Design review of the part built by this model. Coordinates are the model's own, in mm. Coordinates: 2 decimals unless noted, no trailing zeros. Write each loop counter-clockwise with the first axis right and the second up, starting at its lowest first coordinate (ties: lowest second). Pieces come first, ordered by that corner, then holes. Notation, with made-up numbers: (46, 1.5) -> (61, 1.5) arc R31 ccw to (61, 28.5) -> close; hole circle Ø4 at (39.25, -26). An arc over 180 degrees is marked (long way). One line per question, with ' | ' between items. Start each with the question number.
Q1. Wall thickness on probe 1 along X at (y, z) = (87, 77.5); probe 2 along Y at (x, z) = (230, 255): over which ranges is each line inside the solid? List them lowest first.
Q2. Add section C-C on z = 242. State the section outline as (x, y) points.
Q3. For P1, Ø8, axis at y = 140.5, z = -215, coming from the +X side, flat-tipped, find the tip position at first contact; note if it passes through.
Q4. Add section A-A on x = 311.5. State the section outline as (y, z) points.
Q5. Add section D-D on y = 129. State the section outline as (x, z) points, and give its area (3 significant figures).
Q6. Add section B-B on z = 115. State the section outline as (x, y) points, and give its area (3 significant figures).
from build123d import *

# Parameters (mm, degrees)
SKETCH1_W           = 1416.83235241
SKETCH1_H           = 579.478309122
SKETCH1_W_2         = 1270
SKETCH1_H_2         = 434.999892
BOSS_EXTRUDE1_DEPTH = 2.54
SKETCH2_W           = 73.416176205
SKETCH2_H           = 579.478309122
BOSS_EXTRUDE2_DEPTH = 327.9394
SKETCH3_W           = 76.2
SKETCH3_H           = 25.4
BOSS_EXTRUDE3_DEPTH = 299.9994
SKETCH4_W           = 73.416176205
SKETCH4_H           = 579.478309122
BOSS_EXTRUDE4_DEPTH = 149.999954
SKETCH5_W           = 76.2
SKETCH5_H           = 25.4
BOSS_EXTRUDE5_DEPTH = 299.72


with BuildPart() as part:
    # Sketch1 → Boss-Extrude1 (new body)
    with BuildSketch(Plane(origin=(0, 0, 0), x_dir=(1, 0, 0), z_dir=(0, 1, 0))):
        Rectangle(SKETCH1_W, SKETCH1_H)
        Rectangle(SKETCH1_W_2, SKETCH1_H_2, mode=Mode.SUBTRACT)
    extrude(amount=BOSS_EXTRUDE1_DEPTH)

    # Sketch2 → Boss-Extrude2 (add)
    with BuildSketch(Plane.XZ):
        with Locations((-671.708088103, 0)):
            Rectangle(SKETCH2_W, SKETCH2_H)
    extrude(amount=-BOSS_EXTRUDE2_DEPTH)

    # Sketch3 → Boss-Extrude3 (add)
    with BuildSketch(Plane(origin=(-635, 0, 0), x_dir=(0, 0, -1), z_dir=(1, 0, 0))):
        with Locations((-251.639154561, 315.2394)):
            Rectangle(SKETCH3_W, SKETCH3_H)
        with Locations((251.639154561, 315.2394)):
            Rectangle(SKETCH3_W, SKETCH3_H)
    extrude(amount=BOSS_EXTRUDE3_DEPTH)

    # Sketch4 → Boss-Extrude4 (add)
    with BuildSketch(Plane(origin=(0, 327.9394, 0), x_dir=(1, 0, 0), z_dir=(0, 1, 0))):
        with Locations((-671.708088103, 0)):
            Rectangle(SKETCH4_W, SKETCH4_H)
    extrude(amount=BOSS_EXTRUDE4_DEPTH)

    # Sketch5 → Boss-Extrude5 (add)
    with BuildSketch(Plane(origin=(-635, 0, 0), x_dir=(0, 0, -1), z_dir=(1, 0, 0))):
        with Locations((-251.639154561, 465.239354)):
            Rectangle(SKETCH5_W, SKETCH5_H)
        with Locations((251.639154561, 465.239354)):
            Rectangle(SKETCH5_W, SKETCH5_H)
    extrude(amount=BOSS_EXTRUDE5_DEPTH)


solid = part.part
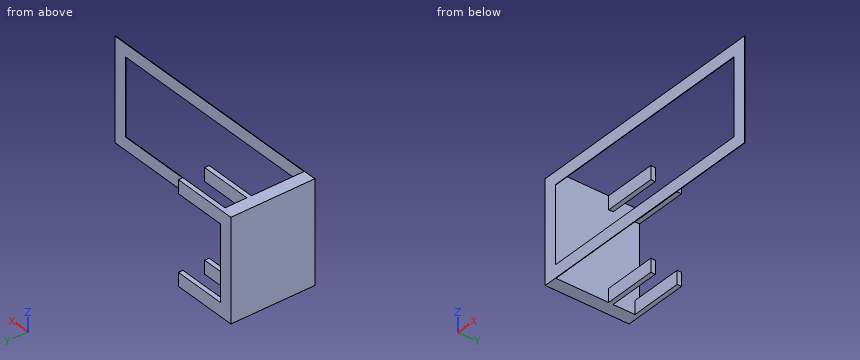
Output values:
1) probe 1: x = -708.42 to -635 | probe 2: y = 0 to 2.54
2) outline: (-708.42, 0) -> (708.42, 0) -> (708.42, 2.54) -> (-635, 2.54) -> (-635, 302.54) -> (-335, 302.54) -> (-335, 327.94) -> (-635, 327.94) -> (-635, 452.54) -> (-335.28, 452.54) -> (-335.28, 477.94) -> (-708.42, 477.94) -> close
3) P1: stops at x = -635
4) outline: (0, -289.74) -> (2.54, -289.74) -> (2.54, -217.5) -> (0, -217.5) -> close; (0, 217.5) -> (2.54, 217.5) -> (2.54, 289.74) -> (0, 289.74) -> close
5) outline: (-708.42, -289.74) -> (-635, -289.74) -> (-635, 289.74) -> (-708.42, 289.74) -> close | area: 42,500 mm2
6) outline: (-708.42, 0) -> (-635, 0) -> (-635, 477.94) -> (-708.42, 477.94) -> close; (635, 0) -> (708.42, 0) -> (708.42, 2.54) -> (635, 2.54) -> close | area: 35,300 mm2
